Part model, mm, in its own coordinate system. A direction names the side the tool comes from. Coordinates: 2 decimals unless noted, no trailing zeros. Order: outer loops, then holes, each group sorted by start corner. A loop starts at its lowest first (then second) coordinate and runs counter-clockwise, first axis right, second up. Notation, with made-up numbers: (76, 42) - (133, 42) arc R20 cw to (133, 49) - close; hole circle Ø4 at (36.5, -14). An arc over 180 degrees is marked (long way). Use a Markdown table: item, result. Add a question column.
1) Drop flat-ended pins along their axis: P1, Ø1.4, axis at x = 41.5, z = 2, coming from the -Y side; P2, Ø0.5, axis at x = 40.5, z = 2, coming from the +Y side; P3, Ø1.5, axis at y = 18.5, z = 6, coming from the +X side. Give the stop position or say it passes through.
2) Two-plate mould, pull along X, no slides. Class faces 1 (the face through (-7.4, 13.5, 5.1)), 2 (the face through (-10.943, 10, 5)), 3 (the face through (39.757, 10, 2)): +X half, -X half, draft (parallel to the pull), parting line (faces both ways), or undercut.
3) Tool access for faces 4 (the face through (-7.3, 6.4, 5.1)), 5 (the face through (42, 9, 2)), 6 (the face through (19.97, 6.504, 5.07)): list every direction of +Z, -Z, +X, -X, +Y, -Y with a clear straight run to the whole face (end or side of a thin tool).
4) Wall check: L1, parallel to Y at x = 4.5, z = 9.25; L2, parallel to Y at x = 40.5, z = 3; L3, parallel to X at y = 1, z = 9. Give the ranges that are in metal, low to high. Write a range as [from, to].
5) Saw through at D-D on y = 12. List the corners of the cut face in (x, z).
6) Saw through at B-B on y = 17.25. List the corners of the cut face in (x, z).
7) Saw through at A-A on x = 4.5. List the corners of the cut face in (y, z), then the cut area to 3 significant figures.
```python
from build123d import *

# Parameters (mm, degrees)
F0_W     = 10.7198789741
F0_H     = 5
F1_DEPTH = 10
F0_W_2   = 2
F0_H_2   = 2
F0_W_3   = 0.7
F2_DEPTH = 4.5
F3_R     = 4.99999
F4_R     = 0.5


# Not quite as in the source:
# - a fillet or chamfer is up to 0.001 mm smaller than in the source, because OpenCascade refuses the exact size


with BuildPart() as f1:
    # F0 (on Top) → F1 (new body)
    with BuildSketch(Plane.XY):
        Polygon((-10.9434188306, 20), (-10.9434188306, 0), (5.6756753474, 0), (5.6756753474, 5), (-8.8288290426, 5), (-8.8288290426, 15), (5.6756753474, 15), (5.6756753474, 20), align=None)
        Polygon((5.6756753474, 5), (5.6756753474, 0), (39.0565811694, 0), (39.0565811694, 7), (39.0565811694, 9), (39.0565811694, 11), (39.0565811694, 13), (39.0565811694, 20), (21.3955543215, 20), (21.3955543215, 15), (21.3955543215, 5), align=None)
        with Locations((11.0356148345, 17.5)):
            Rectangle(F0_W, F0_H)
    extrude(amount=F1_DEPTH)

    # F0 (on Top) → F2 (join)
    with BuildSketch(Plane.XY):
        Polygon((39.0565811694, 9), (39.0565811694, 7), (41.0565811694, 7), (41.0565811694, 9), (39.7565811694, 9), align=None)
        with Locations((42.0565811694, 8)):
            Rectangle(F0_W_2, F0_H_2)
        Polygon((43.0565811694, 7), (41.0565811694, 7), (41.0565811694, 6.25), align=None)
        Polygon((39.0565811694, 13), (39.0565811694, 11), (39.7565811694, 11), (41.0565811694, 11), (41.0565811694, 13), align=None)
        with Locations((42.0565811694, 12)):
            Rectangle(F0_W_2, F0_H_2)
        Polygon((41.0565811694, 13.75), (41.0565811694, 13), (43.0565811694, 13), align=None)
        with Locations((39.4065811694, 10)):
            Rectangle(F0_W_3, F0_H_2)
    extrude(amount=F2_DEPTH)

    # F3 (radius 5 in the source; OpenCascade refuses exactly that, so slightly less here)
    f3_edges = [f1.edges().sort_by_distance(p)[0] for p in [
        (-8.828829, 15, 5),
        (-8.828829, 5, 5),
        (21.395554, 5, 5),
        (21.395554, 20, 5),
    ]]
    fillet(f3_edges, radius=F3_R)

    # F4
    f4_edges = [f1.edges().sort_by_distance(p)[0] for p in [
        (39.056581, 13, 2.25),
        (39.056581, 7, 2.25),
        (41.056581, 7, 2.25),
        (41.056581, 13, 2.25),
        (39.756581, 11, 2.25),
        (39.756581, 9, 2.25),
    ]]
    fillet(f4_edges, radius=F4_R)


solid = f1.part
```
Results are:
| question | item | result |
|---|---|---|
| 1 | P1 | y = 6.25 |
| 1 | P2 | y = 13.04 |
| 1 | P3 | x = 39.06 |
| 2 | face 1 | undercut |
| 2 | face 2 | -X half |
| 2 | face 3 | +X half |
| 3 | face 4 | +Z, -Z |
| 3 | face 5 | +Z, -Z, +X |
| 3 | face 6 | +Z, -Z, +Y |
| 4 | L1 | [0, 5], [15, 20] |
| 4 | L2 | [7, 9], [11, 13] |
| 4 | L3 | [-10.94, 39.06] |
| 5 | outline | (-10.94, 0) - (-8.41, 0) - (-8.41, 10) - (-10.94, 10) - close; (21.4, 0) - (43.06, 0) - (43.06, 4.5) - (39.06, 4.5) - (39.06, 10) - (21.4, 10) - close |
| 6 | outline | (-10.94, 0) - (16.4, 0) - (16.4, 10) - (-10.94, 10) - close; (21.93, 0) - (39.06, 0) - (39.06, 10) - (21.93, 10) - close |
| 7 | outline | (0, 0) - (5, 0) - (5, 10) - (0, 10) - close; (15, 0) - (20, 0) - (20, 10) - (15, 10) - close |
| 7 | area | 100 mm2 |
